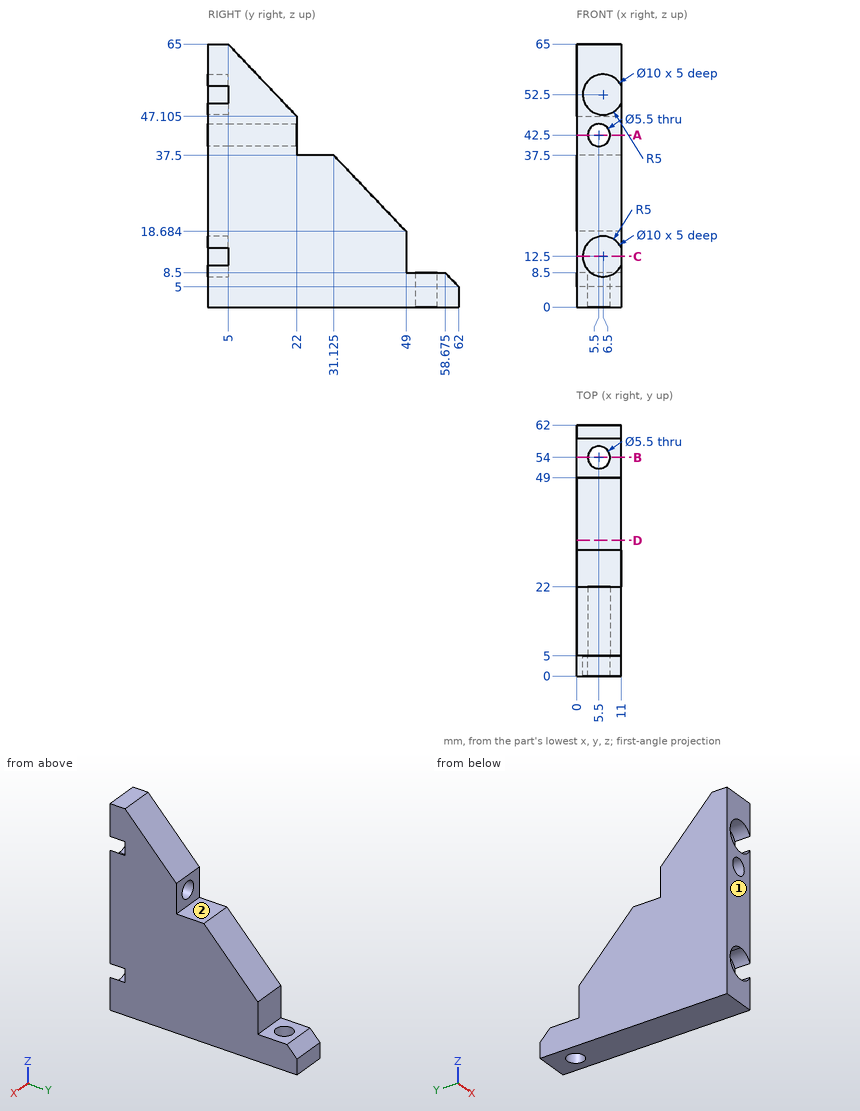
Geometry: see drawing. Coordinates: mm, zero at the bounding-box minimum. A direction names the side the tool comes from. Give positions to 0.01 mm unless a question says otherwise; leave off trailing zeros. Loops run counter-clockwise (first coordinate to the right, second up) from the corner with the lowest first, then second, coordinate; pieces in that order, holes last. Notation, with made-up numbers: (-4, 53.5) - (8, 53.5) arc R16 ccw to (8, 60.5) - close; hole circle Ø6 at (19, -33.75). An arc over 180 degrees is marked (long way). Use CSV: the item, a comma, the result in double quotes. Start each with the question number.
Item 1: Section D-D on y = 33.5. Return loops of the section in (x, z), then the cut area to 3 significant figures.
Item 2: Line query: line 1 (X direction, y = 54, z = 2); line 2 (Z direction, x = 6.5, y = 1.9); line 3 (Y direction, x = 0.5, z = 39). Output: solid intervals per line, ascending.
Item 3: Section A-A on z = 42.5. Return loops of the section in (x, y).
Item 4: Section C-C on z = 12.5. Return loops of the section in (x, y).
Item 5: Contact query for flat-ended pins moving along their axis: P1, Ø1, axis at x = 8, z = 52, coming from the +Y side (1 decimal); P2, Ø3, axis at x = 3.5, y = 53, coming from the +Z side; P3, Ø6, axis at x = 1, y = 51.5, coming from the +Z side; P4, Ø5, axis at x = 5.5, y = 54, coming from the -Z side. Output: stop coordinate, or through.
Item 6: Section B-B on y = 54. Return loops of the section in (x, z).
Item 7: Reachability of the marked faces 1 and 2 from +Z, -Z, +X, -X, +Y, -Y: full face, straight path, thin tool, end or side. Return the list, or none.
Ans:
1,outline,"(0, 0) - (11, 0) - (11, 35) - (0, 35) - close"
1,area,"385 mm2"
2,line 1,"x = 0 to 2.75, 8.25 to 11"
2,line 2,"z = 0 to 7.5, 17.5 to 39.94, 45.06 to 47.5, 57.5 to 65"
2,line 3,"y = 0 to 22"
3,outline,"(0, 0) - (2.75, 0) - (2.75, 22) - (0, 22) - close; (8.25, 0) - (11, 0) - (11, 22) - (8.25, 22) - close"
4,outline,"(0, 0) - (1.5, 0) - (1.5, 5) - (11, 5) - (11, 49) - (0, 49) - close"
5,P1,"stops at y = 17.8"
5,P2,"stops at z = 8.5"
5,P3,"stops at z = 19.21"
5,P4,"passes through"
6,outline,"(0, 0) - (2.75, 0) - (2.75, 8.5) - (0, 8.5) - close; (8.25, 0) - (11, 0) - (11, 8.5) - (8.25, 8.5) - close"
7,face 1,"+Z, -Z, +X, -X, -Y"
7,face 2,"+Z, +X, -X, +Y"
